from build123d import *
from build123d.topology import SkipClean

# Parameters (mm, degrees)
SKETCH5_W           = 10.3
SKETCH5_H           = 10.3
BOSS_EXTRUDE2_DEPTH = 4.6
SKETCH6_W           = 8.3
SKETCH6_H           = 2.6
CUT_EXTRUDE3_DEPTH  = 9.3
BOSS_EXTRUDE4_DEPTH = 1.1
BOSS_EXTRUDE5_REACH = 12.83
SKETCH10_R          = 2
CUT_EXTRUDE4_DEPTH  = 12.234169035
SKETCH11_R          = 3.1
SKETCH11_R_2        = 2
BOSS_EXTRUDE6_DEPTH = 1.7
SKETCH12_R          = 4
BOSS_EXTRUDE7_DEPTH = 1.2
BOSS_EXTRUDE8_DEPTH = 0.6
CUT_EXTRUDE7_DEPTH  = 14.165903481
CUT_EXTRUDE8_DEPTH  = 13.784307824
SKETCH16_R          = 6.11839758
SKETCH16_R_2        = 4.91839758
BOSS_EXTRUDE9_DEPTH = 1.2
CUT_EXTRUDE9_START  = -1.2
CUT_EXTRUDE9_DEPTH  = 1.2


with BuildPart() as part:
    # Sketch5 → Boss-Extrude2 (new body)
    with BuildSketch(Plane(origin=(0, 0, 0), x_dir=(1, 0, 0), z_dir=(0, 1, 0))):
        with Locations((0.148353909, 1.208024691)):
            Rectangle(SKETCH5_W, SKETCH5_H)
    extrude(amount=BOSS_EXTRUDE2_DEPTH)

    # Sketch6 → Cut-Extrude3 (cut)
    with BuildSketch(Plane(origin=(5.298353909, 0, 0), x_dir=(0, 0, -1), z_dir=(1, 0, 0))):
        with Locations((1.208024691, 2.3)):
            Rectangle(SKETCH6_W, SKETCH6_H)
    cut_extrude3 = extrude(amount=-CUT_EXTRUDE3_DEPTH, mode=Mode.SUBTRACT)

    # Sketch7 → Boss-Extrude4 (add)
    with BuildSketch(Plane(origin=(0, 4.6, 0), x_dir=(1, 0, 0), z_dir=(0, 1, 0))):
        with BuildLine():
            Line((4.049956144, 7.358024691), (-3.753248326, 7.358024691))
            ThreePointArc((-3.753248326, 7.358024691), (-4.404982862, 6.89240014), (-5.001646091, 6.358024691))
            Line((-5.001646091, 6.358024691), (5.298353909, 6.358024691))
            ThreePointArc((5.298353909, 6.358024691), (4.701690681, 6.89240014), (4.049956144, 7.358024691))
        make_face()
        with BuildLine():
            Line((-5.001646091, -3.941975309), (-5.001646091, 6.358024691))
            ThreePointArc((-5.001646091, 6.358024691), (-7.134845937, 1.208024691), (-5.001646091, -3.941975309))
        make_face()
        with BuildLine():
            Line((5.298353909, -3.941975309), (-5.001646091, -3.941975309))
            ThreePointArc((-5.001646091, -3.941975309), (-4.404982862, -4.476350758), (-3.753248326, -4.941975309))
            Line((-3.753248326, -4.941975309), (4.049956144, -4.941975309))
            ThreePointArc((4.049956144, -4.941975309), (4.701690681, -4.476350758), (5.298353909, -3.941975309))
        make_face()
        with BuildLine():
            ThreePointArc((5.298353909, -1.787660692), (6.106258819, 1.208024691), (5.298353909, 4.203710075))
            Line((5.298353909, 4.203710075), (5.298353909, -1.787660692))
        make_face()
    boss_extrude4 = extrude(amount=-BOSS_EXTRUDE4_DEPTH)

    # Mirror1: Cut-Extrude3, Boss-Extrude4 across plane
    add(cut_extrude3.mirror(Plane.ZX.offset(2.3)), mode=Mode.SUBTRACT)
    add(boss_extrude4.mirror(Plane.ZX.offset(2.3)))

    # Sketch8 → Boss-Extrude5 (add, up to next)
    with BuildSketch(Plane(origin=(0, 1.1, 0), x_dir=(1, 0, 0), z_dir=(0, 1, 0)), mode=Mode.PRIVATE) as boss_extrude5_sk1:
        with BuildLine():
            Line((-6.334845937, 4.52662677), (-6.334845937, -2.110577387))
            ThreePointArc((-6.334845937, -2.110577387), (-5.739883454, -3.078426142), (-5.001646091, -3.941975309))
            Line((-5.001646091, -3.941975309), (-5.001646091, 6.358024691))
            ThreePointArc((-5.001646091, 6.358024691), (-5.739883454, 5.494475525), (-6.334845937, 4.52662677))
        make_face()
    boss_extrude5_tool1 = extrude(boss_extrude5_sk1.sketch, amount=BOSS_EXTRUDE5_REACH, mode=Mode.PRIVATE) - part.part
    add(boss_extrude5_tool1.solids().sort_by_distance((-5.621972, 1.1, -1.208025))[0])

    # Sketch10 → Cut-Extrude4 (cut, through all)
    with SkipClean():  # the faces are left unmerged after this step: merging them gives an invalid solid
        with BuildSketch(Plane.XZ):
            with Locations(Location((-0.514293559, -1.208024691, 0), (0, 0, 270))):
                Circle(SKETCH10_R)
        extrude(amount=-CUT_EXTRUDE4_DEPTH, mode=Mode.SUBTRACT)

    # Sketch11 → Boss-Extrude6 (add)
    with SkipClean():  # the faces are left unmerged after this step: merging them gives an invalid solid
        with BuildSketch(Plane(origin=(0, 4.6, 0), x_dir=(1, 0, 0), z_dir=(0, 1, 0))):
            with Locations(Location((-0.514293559, 1.208024691, 0), (0, 0, 90))):
                Circle(SKETCH11_R)
            with Locations(Location((-0.514293559, 1.208024691, 0), (0, 0, 90))):
                Circle(SKETCH11_R_2, mode=Mode.SUBTRACT)
        extrude(amount=BOSS_EXTRUDE6_DEPTH)

    # Sketch12 → Boss-Extrude7 (add)
    with SkipClean():  # the faces are left unmerged after this step: merging them gives an invalid solid
        with BuildSketch(Plane(origin=(0, 6.3, 0), x_dir=(1, 0, 0), z_dir=(0, 1, 0))):
            with Locations(Location((-0.514293559, 1.208024691, 0), (0, 0, 270))):
                Circle(SKETCH12_R)
        extrude(amount=BOSS_EXTRUDE7_DEPTH)

    # Sketch13 → Boss-Extrude8 (add)
    with SkipClean():  # the faces are left unmerged after this step: merging them gives an invalid solid
        with BuildSketch(Plane(origin=(0, 7.5, 0), x_dir=(1, 0, 0), z_dir=(0, 1, 0))):
            with BuildLine():
                Line((-1.214293559, 5.146298425), (-1.214293559, 1.908024691))
                Line((-1.214293559, 1.908024691), (-4.452567292, 1.908024691))
                ThreePointArc((-4.452567292, 1.908024691), (-4.514293559, 1.208024691), (-4.452567292, 0.508024691))
                Line((-4.452567292, 0.508024691), (-1.214293559, 0.508024691))
                Line((-1.214293559, 0.508024691), (-1.214293559, -2.730249042))
                ThreePointArc((-1.214293559, -2.730249042), (-0.514293559, -2.791975309), (0.185706441, -2.730249042))
                Line((0.185706441, -2.730249042), (0.185706441, 0.508024691))
                Line((0.185706441, 0.508024691), (3.423980175, 0.508024691))
                ThreePointArc((3.423980175, 0.508024691), (3.485706441, 1.208024691), (3.423980175, 1.908024691))
                Line((3.423980175, 1.908024691), (0.185706441, 1.908024691))
                Line((0.185706441, 1.908024691), (0.185706441, 5.146298425))
                ThreePointArc((0.185706441, 5.146298425), (-0.514293559, 5.208024691), (-1.214293559, 5.146298425))
            make_face()
        extrude(amount=BOSS_EXTRUDE8_DEPTH)

    # Sketch14 → Cut-Extrude7 (cut, through all)
    with SkipClean():  # the faces are left unmerged after this step: merging them gives an invalid solid
        with BuildSketch(Plane(origin=(0.185706441, 0, 0), x_dir=(0, 0, -1), z_dir=(1, 0, 0))):
            Polygon((-2.8486475, 7.5), (0.508024691, 8.1), (-2.8486475, 8.1), align=None)
            Polygon((5.264696882, 7.5), (1.908024691, 8.1), (5.264696882, 8.1), align=None)
        extrude(amount=-CUT_EXTRUDE7_DEPTH, mode=Mode.SUBTRACT)

    # Sketch15 → Cut-Extrude8 (cut, through all)
    with SkipClean():  # the faces are left unmerged after this step: merging them gives an invalid solid
        with BuildSketch(Plane.XY.offset(-0.508024691)):
            Polygon((3.521468612, 8.1), (3.521468612, 7.5), (0.185706441, 8.1), align=None)
            Polygon((-4.550055729, 7.5), (-1.214293559, 8.1), (-4.550055729, 8.1), align=None)
        extrude(amount=-CUT_EXTRUDE8_DEPTH, mode=Mode.SUBTRACT)

    # Sketch16 → Boss-Extrude9 (add)
    with SkipClean():  # the faces are left unmerged after this step: merging them gives an invalid solid
        with BuildSketch(Plane.XZ):
            with Locations(Location((-0.514293559, -1.208024691, 0), (0, 0, 270))):
                Circle(SKETCH16_R)
            with Locations(Location((-0.514293559, -1.208024691, 0), (0, 0, 270))):
                Circle(SKETCH16_R_2, mode=Mode.SUBTRACT)
        extrude(amount=BOSS_EXTRUDE9_DEPTH)

    # Sketch17 → Cut-Extrude9 (cut)
    with SkipClean():  # the faces are left unmerged after this step: merging them gives an invalid solid
        with BuildSketch(Plane.XZ.offset(1.2).offset(CUT_EXTRUDE9_START)):
            with BuildLine():
                Line((3.364577542, 1.816044378), (3.364577542, -4.232093761))
                Line((3.364577542, -4.232093761), (3.415683395, -5.897381799))
                ThreePointArc((3.415683395, -5.897381799), (5.604014001, -1.174835129), (3.364577542, 3.523692537))
                Line((3.364577542, 3.523692537), (3.364577542, 1.816044378))
            make_face()
        extrude(amount=CUT_EXTRUDE9_DEPTH, mode=Mode.SUBTRACT)


solid = part.part
For this review, take the finished solid that the model builds, in its own axes (mm). A direction names the side the tool comes from. Round coordinates to 2 decimals unless told otherwise and drop trailing zeros. Loops run counter-clockwise (first coordinate to the right, second up) from the corner with the lowest first, then second, coordinate; pieces in that order, holes last. Notation, with made-up numbers: (87.5, -28.75) - (101.5, -28.75) arc R20 cw to (101.5, -5.75) - close; hole circle Ø4 at (36, -21). An arc over 180 degrees is marked (long way). Answer as CSV lines item,"result".
(1) Consider section B-B on x = 5. Give the boundary of the cut face in (y, z), then the cut area to 3 significant figures.
Checked values:
outline,"(0, -6.64) - (1.1, -6.64) - (1.1, -6.36) - (3.5, -6.36) - (3.5, -6.64) - (4.6, -6.64) - (4.6, 4.22) - (3.5, 4.22) - (3.5, 3.94) - (1.1, 3.94) - (1.1, 4.22) - (0, 4.22) - close; hole (1, -5.36) - (3.6, -5.36) - (3.6, 2.94) - (1, 2.94) - close"
area,"27.0 mm2"
(2) Consider section D-D on y = 5.25. Give the boundary of the cut face in (x, z).
Checked values:
outline,"circle Ø6.2 at (-0.51, -1.21); hole circle Ø4 at (-0.51, -1.21)"
(3) Insertion check: P1, Ø2.5, axis at x = -2.5, z = -4, coming from the +Y side; P2, Ø3, axis at y = 5, z = 1.5, coming from the +X side; P3, Ø0.7, axis at x = 4, z = 0.5, coming from the -Y side. Each pin has a flat end and moves straight along its axis. Give the tip position at first contact, or say it passes through.
Checked values:
P1,"stops at y = 7.5"
P2,"stops at x = 5.97"
P3,"stops at y = 0"
(4) Consider section A-A on y = 2.25. Give the boundary of the cut face in (x, z), then the cut area to 3 significant figures.
Checked values:
outline,"(-6.33, -4.53) arc R7.28 ccw to (-5, -6.36) - (5.3, -6.36) - (5.3, -5.36) - (-4, -5.36) - (-4, 2.94) - (5.3, 2.94) - (5.3, 3.94) - (-5, 3.94) arc R7.28 ccw to (-6.33, 2.11) - close"
area,"40.5 mm2"
(5) Tool access review of faces 1 (the face through (-3, 6.3, 1)), 2 (the face through (0.1, 3.5, 4.4)), 3 (the face through (3.365, -1, 3)), 4 (the face through (-2, 7.5, 1)), 5 (the face through (-1.42, 6.9, 2.69)): name each direction out of +Z, -Z, +X, -X, +Y, -Y from which nothing blocks a thin tool from reaching the whole face with its end or side.
Checked values:
face 1,"none"
face 2,"+Z, +X, -X"
face 3,"+Z, +X, -Y"
face 4,"+Z, -X, +Y"
face 5,"+Y"
(6) Mouldability with a two-part tool opening along Z and no side actions: class faces 6 (the face through (6.106, 0.542, -1.164)), 7 (the face through (-0.43, 0.49, 0.79)), 8 (the face through (5.298, 2.3, 3.1)) as +Z half, -Z half, draft (parallel to the pull), parting line (faces both ways), or undercut.
Checked values:
face 6,"parting line"
face 7,"undercut"
face 8,"draft"
(7) Wall thickness on line 1 (Y direction, x = 2.5, z = -3.75); line 2 (Z direction, x = -0.25, y = 2.5); line 3 (Y direction, x = 1, z = 0.75): over which ranges is each line inside the solid? List them lowest first.
Checked values:
line 1,"y = 0 to 1, 3.6 to 4.6, 6.3 to 7.5"
line 2,"z = -6.36 to -5.36, 2.94 to 3.94"
line 3,"y = 0 to 1, 3.6 to 7.5"
